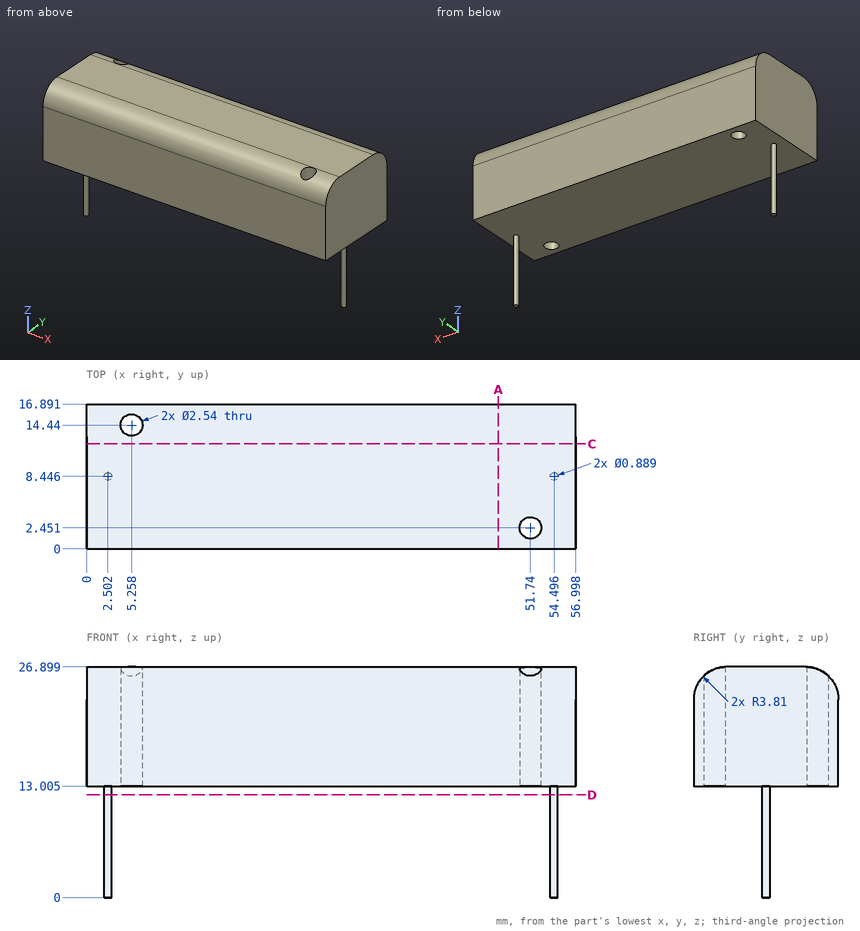
Geometry: see drawing. Coordinates: mm, zero at the bounding-box minimum. Give positions to 0.01 mm unless a question says otherwise; leave off trailing zeros. Write each loop counter-clockwise with the first axis right and the second up, starting at its lowest first coordinate (ties: lowest second). Pieces come first, ordered by that corner, then holes. Notation, with made-up numbers: (62, 36.5) -> (91, 36.5) arc R23 cw to (91, 68.5) -> close; hole circle Ø5 at (63.5, -21.5). An arc over 180 degrees is marked (long way). Use one line per item in the form item = value. Start each with the question number.
1) Section query C-C on y = 12.25. Return the cut outline in (x, z) (1 decimal).
2) Ray query, probe 1 along Z at (x, y) = (22.5, 6) (1 decimal); probe 2 along Y at (x, z) = (36, 25.75) (1 decimal); probe 3 along Y at (x, z) = (54, 23.75). Return the intervals inside material, ascending. Write a range as from..to.
3) Pin query (flat end, axial travel): pin 1 (10 mm diameter, centred on x = 31, y = 14, fed in from -Z) (1 decimal); pin 2 (5 mm diameter, centred on y = 5, z = 7.5, fed in from +X). Return the tip coordinate at first contact, or that it passes through.
4) Section query D-D on z = 12. Return the cut outline in (x, y) (1 decimal).
5) Section query A-A on x = 48. Return the cut outline in (y, z) (1 decimal).
Outcome:
q1.outline = (0, 13) -> (57, 13) -> (57, 26.9) -> (0, 26.9) -> close
q2.probe_1 = 13..26.9
q2.probe_2 = 1.1..15.8
q2.probe_3 = 0.06..16.83
q3.pin_1 = 13
q3.pin_2 = through
q4.outline = circle Ø0.9 at (2.5, 8.4); circle Ø0.9 at (54.5, 8.4)
q5.outline = (0, 13) -> (16.9, 13) -> (16.9, 23.1) arc R3.8 ccw to (13.1, 26.9) -> (3.8, 26.9) arc R3.8 ccw to (0, 23.1) -> close
